CAD build for the part. Positions are in the model's coordinates, mm. A direction names the side the tool comes from. Give positions to 0.01 mm unless a question says otherwise; leave off trailing zeros. Loops run counter-clockwise (first coordinate to the right, second up) from the corner with the lowest first, then second, coordinate; pieces in that order, holes last. Notation, with made-up numbers: M 11.25,-30.5 L 19.25,-30.5 A7 cw 19.25,-22.5 Z; hole C 9,-37.75 d9. An arc over 180 degrees is marked long. One line per question, with ' | ' between items.
```python
from build123d import *

# Parameters (mm, degrees)
ESQUISSE1_R             = 12
BOSS_EXTRU_1_DEPTH      = 2.5
ESQUISSE2_R             = 5
ESQUISSE2_R_2           = 2.75
BOSS_EXTRU_2_DEPTH      = 3.6
ESQUISSE3_R             = 1.490305946
ESQUISSE3_R_2           = 1.25
ENL_V_MAT_EXTRU_1_DEPTH = 19.033579789


with BuildPart() as part:
    # Esquisse1 → Boss.-Extru.1 (new body)
    with BuildSketch(Plane.XY):
        Circle(ESQUISSE1_R)
    extrude(amount=BOSS_EXTRU_1_DEPTH)

    # Esquisse2 → Boss.-Extru.2 (add)
    with BuildSketch(Plane.XY.offset(2.5)):
        Circle(ESQUISSE2_R)
        Circle(ESQUISSE2_R_2, mode=Mode.SUBTRACT)
    extrude(amount=BOSS_EXTRU_2_DEPTH)

    # Esquisse3 → Enlèv. mat.-Extru.1 (cut, through all)
    with BuildSketch(Plane(origin=(0, 0, 0), x_dir=(-1, 0, 0), z_dir=(0, 0, -1))):
        Circle(ESQUISSE3_R)
        with Locations((0, 8.5)):
            Circle(ESQUISSE3_R_2)
        with Locations((8.5, 0)):
            Circle(ESQUISSE3_R_2)
        with Locations((0, -8.5)):
            Circle(ESQUISSE3_R_2)
        with Locations((-8.5, 0)):
            Circle(ESQUISSE3_R_2)
    extrude(amount=-ENL_V_MAT_EXTRU_1_DEPTH, mode=Mode.SUBTRACT)


solid = part.part
```
Item 1: Drill centre lines: line 1 along Y through (x, z) = (0, 1.2); line 2 along Y through (x, z) = (-0.5, 1.25); line 3 along X through (y, z) = (-8.75, 1). Where is each one in solid material? Low to high. Write a range as [from, to].
Conclusion:
line 1: [-12, -9.75], [-7.25, -1.49], [1.49, 7.25], [9.75, 12] | line 2: [-11.99, -9.65], [-7.35, -1.4], [1.4, 7.35], [9.65, 11.99] | line 3: [-8.21, -1.22], [1.22, 8.21]
Item 2: Mould opens along Y. For faces 3 (the cylindrical face through (-11.99, 0.53, 1.23)), 4 (the flat face through (1.2, -1.2, 2.5)), 5 (the flat face through (2.2, -2.2, 6.1)) say: pulls with the +Y half, pulls with the -Y half, needs draft (parallel to the pull), parting line crosses it, or undercut.
Conclusion:
face 3: parting line crosses it | face 4: undercut | face 5: needs draft
Item 3: Drop flat-ended pins along their axis: P1, Ø1, axis at x = -0.5, y = -7.5, coming from the +Z side; P2, Ø2, axis at y = -1, z = 4, coming from the -X side. Give the stop position or say it passes through.
Conclusion:
P1: z = 2.5 | P2: x = -5
Item 4: Saw through at C-C on y = -8.5. Give the cut face in (x, z).
Conclusion:
outline: M -8.47,0 L -1.25,0 L -1.25,2.5 L -8.47,2.5 Z; M 1.25,0 L 8.47,0 L 8.47,2.5 L 1.25,2.5 Z
Item 5: 3-axis set-ups, long thin cutter, end or side, ignore diameter. For faces 1 (the flat face through (5.2, 0.2, 2.5)), 2 (the cylindrical face through (-7.25, 0.05, 1.23)): which of +Z, -Z, +X, -X, +Y, -Y reach the whole face in a straight line?
Conclusion:
face 1: +Z | face 2: +Z, -Z
Item 6: Saw through at A-A on y = 0. Give the cut face in (x, z).
Conclusion:
outline: M -12,0 L -9.75,0 L -9.75,2.5 L -12,2.5 Z; M -7.25,0 L -1.49,0 L -1.49,2.5 L -2.75,2.5 L -2.75,6.1 L -5,6.1 L -5,2.5 L -7.25,2.5 Z; M 1.49,0 L 7.25,0 L 7.25,2.5 L 5,2.5 L 5,6.1 L 2.75,6.1 L 2.75,2.5 L 1.49,2.5 Z; M 9.75,0 L 12,0 L 12,2.5 L 9.75,2.5 Z
